```python
from build123d import *

# Parameters (mm, degrees)
SKETCH1_W           = 46
SKETCH1_H           = 32
BOSS_EXTRUDE1_DEPTH = 21.5
SKETCH2_R           = 4
SKETCH2_R_2         = 1.5
BOSS_EXTRUDE2_DEPTH = 2
FILLET1_R           = 3
FILLET2_R           = 3
SKETCH3_R           = 3
BOSS_EXTRUDE3_DEPTH = 15.7
CUT_EXTRUDE1_START  = -10
CUT_EXTRUDE1_DEPTH  = 10
SKETCH6_R           = 6
BOSS_EXTRUDE4_DEPTH = 2
SKETCH7_R           = 12.2
BOSS_EXTRUDE5_DEPTH = 31
SKETCH8_W           = 1.14055435
SKETCH8_H           = 4.159430758
BOSS_EXTRUDE6_DEPTH = 8
CHAMFER1_SIZE       = 0.8
CHAMFER2_SIZE       = 0.8
SKETCH9_R           = 1
CUT_EXTRUDE2_DEPTH  = 8
SKETCH10_R          = 4
BOSS_EXTRUDE7_DEPTH = 2
FILLET3_R           = 0.2
FILLET4_R           = 0.2
FILLET5_R           = 0.2
FILLET6_R           = 0.2
FILLET7_R           = 0.3
SCALE3_SCALE        = 0.6


with BuildPart() as part:
    # Sketch1 → Boss-Extrude1 (new body)
    with BuildSketch(Plane(origin=(0, 0, 0), x_dir=(1, 0, 0), z_dir=(0, 1, 0))):
        with Locations((23, 16)):
            Rectangle(SKETCH1_W, SKETCH1_H)
    extrude(amount=BOSS_EXTRUDE1_DEPTH)

    # Sketch2 → Boss-Extrude2 (add)
    # profile 1 of 4: a face of its own
    with BuildSketch(Plane(origin=(0, 21.5, 0), x_dir=(1, 0, 0), z_dir=(0, 1, 0))):
        with Locations(Location((6.5, 25, 0), (0, 0, 90))):
            Circle(SKETCH2_R)
        with Locations(Location((6.5, 25, 0), (0, 0, 270))):
            Circle(SKETCH2_R_2, mode=Mode.SUBTRACT)
    # profile 2 of 4: a face of its own
    with BuildSketch(Plane(origin=(0, 21.5, 0), x_dir=(1, 0, 0), z_dir=(0, 1, 0))):
        with Locations(Location((39.5, 25, 0), (0, 0, 90))):
            Circle(SKETCH2_R)
        with Locations(Location((39.5, 25, 0), (0, 0, 270))):
            Circle(SKETCH2_R_2, mode=Mode.SUBTRACT)
    # profile 3 of 4: a face of its own
    with BuildSketch(Plane(origin=(0, 21.5, 0), x_dir=(1, 0, 0), z_dir=(0, 1, 0))):
        with Locations(Location((39.5, 7, 0), (0, 0, 90))):
            Circle(SKETCH2_R)
        with Locations(Location((39.5, 7, 0), (0, 0, 90))):
            Circle(SKETCH2_R_2, mode=Mode.SUBTRACT)
    # profile 4 of 4: a face of its own
    with BuildSketch(Plane(origin=(0, 21.5, 0), x_dir=(1, 0, 0), z_dir=(0, 1, 0))):
        with Locations(Location((6.5, 7, 0), (0, 0, 90))):
            Circle(SKETCH2_R)
        with Locations(Location((6.5, 7, 0), (0, 0, 90))):
            Circle(SKETCH2_R_2, mode=Mode.SUBTRACT)
    extrude(amount=BOSS_EXTRUDE2_DEPTH)

    # Fillet1
    fillet1_edges = [part.edges().sort_by_distance(p)[0] for p in [
        (46, 10.75, -32),
    ]]
    fillet(fillet1_edges, radius=FILLET1_R)

    # Fillet2
    fillet2_edges = [part.edges().sort_by_distance(p)[0] for p in [
        (0, 10.75, -32),
        (46, 10.75, 0),
        (0, 10.75, 0),
    ]]
    fillet(fillet2_edges, radius=FILLET2_R)

    # Sketch3 → Boss-Extrude3 (add)
    with BuildSketch(Plane(origin=(0, 21.5, 0), x_dir=(1, 0, 0), z_dir=(0, 1, 0))):
        with Locations(Location((15.5, 16, 0), (0, 0, 90))):
            Circle(SKETCH3_R)
    extrude(amount=BOSS_EXTRUDE3_DEPTH)

    # Sketch5 → Cut-Extrude1 (cut)
    with BuildSketch(Plane(origin=(0, 37.2, 0), x_dir=(1, 0, 0), z_dir=(0, 1, 0)).offset(CUT_EXTRUDE1_START)):
        with BuildLine():
            Line((17, 18.598076211), (17, 13.401923789))
            ThreePointArc((17, 13.401923789), (18.5, 16), (17, 18.598076211))
        make_face()
    extrude(amount=CUT_EXTRUDE1_DEPTH, mode=Mode.SUBTRACT)

    # Sketch6 → Boss-Extrude4 (add)
    with BuildSketch(Plane(origin=(0, 21.5, 0), x_dir=(1, 0, 0), z_dir=(0, 1, 0))):
        with Locations(Location((15.5, 16, 0), (0, 0, 90))):
            Circle(SKETCH6_R)
    extrude(amount=BOSS_EXTRUDE4_DEPTH)

    # Sketch7 → Boss-Extrude5 (add)
    with BuildSketch(Plane(origin=(46, 0, 0), x_dir=(0, 0, -1), z_dir=(1, 0, 0))):
        with Locations(Location((16, 9, 0), (0, 0, 227.536275048))):
            Circle(SKETCH7_R)
    extrude(amount=BOSS_EXTRUDE5_DEPTH)

    # Sketch8 → Boss-Extrude6 (add)
    with BuildSketch(Plane(origin=(77, 0, 0), x_dir=(0, 0, -1), z_dir=(1, 0, 0))):
        with Locations((16, 17.5)):
            Rectangle(SKETCH8_W, SKETCH8_H)
        with Locations((16, 0.5)):
            Rectangle(SKETCH8_W, SKETCH8_H)
    extrude(amount=BOSS_EXTRUDE6_DEPTH)

    # Chamfer1
    chamfer1_edges = [part.edges().sort_by_distance(p)[0] for p in [
        (85, 19.579715379, -16),
    ]]
    chamfer(chamfer1_edges, length=CHAMFER1_SIZE)

    # Chamfer2
    chamfer2_edges = [part.edges().sort_by_distance(p)[0] for p in [
        (85, -1.579715379, -16),
        (85, 2.579715379, -16),
        (85, 15.420284621, -16),
    ]]
    chamfer(chamfer2_edges, length=CHAMFER2_SIZE)

    # Sketch9 → Cut-Extrude2 (cut)
    with BuildSketch(Plane.XY.offset(-15.429722825)):
        with Locations((82, 17.5)):
            Circle(SKETCH9_R)
        with Locations((82, 0.5)):
            Circle(SKETCH9_R)
    extrude(amount=-CUT_EXTRUDE2_DEPTH, mode=Mode.SUBTRACT)

    # Sketch10 → Boss-Extrude7 (add)
    with BuildSketch(Plane(origin=(0, 21.5, 0), x_dir=(1, 0, 0), z_dir=(0, 1, 0))):
        with Locations(Location((28.5, 22, 0), (0, 0, 90))):
            Circle(SKETCH10_R)
        with Locations(Location((28.5, 10, 0), (0, 0, 90))):
            Circle(SKETCH10_R)
    extrude(amount=BOSS_EXTRUDE7_DEPTH)

    # Fillet3
    fillet3_edges = [part.edges().sort_by_distance(p)[0] for p in [
        (28.5, 23.5, -6),
    ]]
    fillet(fillet3_edges, radius=FILLET3_R)

    # Fillet4
    fillet4_edges = [part.edges().sort_by_distance(p)[0] for p in [
        (28.5, 23.5, -18),
    ]]
    fillet(fillet4_edges, radius=FILLET4_R)

    # Fillet5
    fillet5_edges = [part.edges().sort_by_distance(p)[0] for p in [
        (12.602222521, 37.2, -15.223542865),
    ]]
    fillet(fillet5_edges, radius=FILLET5_R)

    # Fillet6
    fillet6_edges = [part.edges().sort_by_distance(p)[0] for p in [
        (77, 18, -24.236504113),
    ]]
    fillet(fillet6_edges, radius=FILLET6_R)

    # Fillet7
    # the kernel refuses this fillet: 0.3 mm, written as the material it takes off along each edge
    with BuildSketch(Plane(origin=(46, 9, -16), x_dir=(0, -0.6948182221031018, 0.7191853990686162), z_dir=(0, 0.7191853990686162, 0.6948182221031018))) as fillet7_piece_1_section:
        with BuildLine():
            CenterArc((12.2 - FILLET7_R, FILLET7_R), FILLET7_R, 270, 90)
            Line((12.2 - FILLET7_R, 0), (12.2, 0))
            Line((12.2, 0), (12.2, FILLET7_R))
        make_face()
    fillet7_piece_1 = revolve(axis=Axis((46, 9, -16), (1, 0, 0)), revolution_arc=91.974532738, mode=Mode.PRIVATE)
    fillet7_piece_1 = split(fillet7_piece_1, bisect_by=Plane(origin=(46.082910909, 0, -16), z_dir=(0, -1, 0)), keep=Keep.TOP, mode=Mode.PRIVATE)
    add(fillet7_piece_1, mode=Mode.SUBTRACT)


with BuildPart() as part_1:
    # Scale3: scaled about (34.850364497, 10.537899591, -15.999999996)
    add(part.part.scale(SCALE3_SCALE).moved(Location((13.940145799, 4.215159836, -6.399999998))))


solid = part_1.part
```
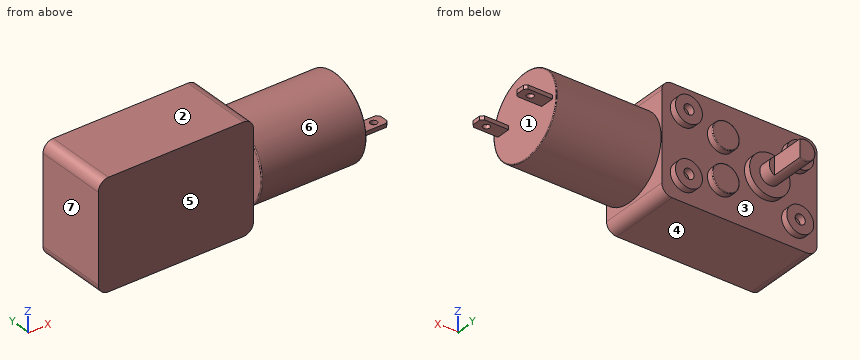
The model under review builds one solid part; all positions refer to its coordinate system, in mm. Face numbers are marked on the shaded views. A direction names the side the tool comes from. Round coordinates to 2 decimals unless told otherwise and drop trailing zeros. Loops run counter-clockwise (first coordinate to the right, second up) from the corner with the lowest first, then second, coordinate; pieces in that order, holes last. Notation, with made-up numbers: (-2, 58) - (49, 58) arc R14 cw to (49, 81) - close; hole circle Ø1 at (-25, -14.75). An arc over 180 degrees is marked (long way). Use a Markdown table: item, result. Add a question column.
Q1. The part is to be moulded in two halves that separate along Z. For the marked faces 1, 2, 3 and 4, say which applies: pulls with the +Z half, pulls with the -Z half, needs draft (parallel to the pull), parting line crosses it, or undercut.
Q2. Machinability: for the marked faces 5, 6 and 7, which of the approach directions +Z, -Z, +X, -X, +Y, -Y give a long, thin tool a straight path to every point of the face, cutting with its end or side? Answer none if there is none.
Q3. Insertion check: pin 1 Ø5.5 at (x, z) = (18, -10.5) entering from +Y; pin 2 Ø4 at (y, z) = (7, -10.5) entering from +X; pin 3 Ø0.9 at (y, z) = (3.5, -17.5) entering from -X. Each pin has a flat end and moves straight along its axis. Give the tip position at first contact, or say it passes through.
Q4. Add section A-A (x = 53). State the section outline as (y, z) points.
Q5. For probe 1 along X at (y, z) = (17.5, -10.6); probe 2 along X at (y, z) = (11.5, -17.5); probe 3 along X at (y, z) = (12.5, -8.5), list the stretches that pass through material, from the lowest coordinate up.
Q6. Add section B-B (y = 19). State the section outline as (x, z) points, plus the area to 3 significant figures.
Worked answers:
| question | item | result |
|---|---|---|
| 1 | face 1 | needs draft |
| 1 | face 2 | pulls with the +Z half |
| 1 | face 3 | undercut |
| 1 | face 4 | pulls with the -Z half |
| 2 | face 5 | +Z, -Z, -X, -Y |
| 2 | face 6 | +X |
| 2 | face 7 | +Z, -Z, -X, +Y, -Y |
| 3 | pin 1 | y = 18.32 |
| 3 | pin 2 | x = 60.14 |
| 3 | pin 3 | x = 41.54 |
| 4 | outline | circle Ø14.64 at (9.62, -16) |
| 5 | probe 1 | 15.44 to 16.94, 18.74 to 20.24, 29.45 to 32.63, 35.24 to 36.74, 38.54 to 40.04 |
| 5 | probe 2 | 13.94 to 60.14 |
| 5 | probe 3 | 13.94 to 41.54 |
| 6 | outline | circle Ø3.6 at (23.24, -16) |
| 6 | area | 10.2 mm² |
